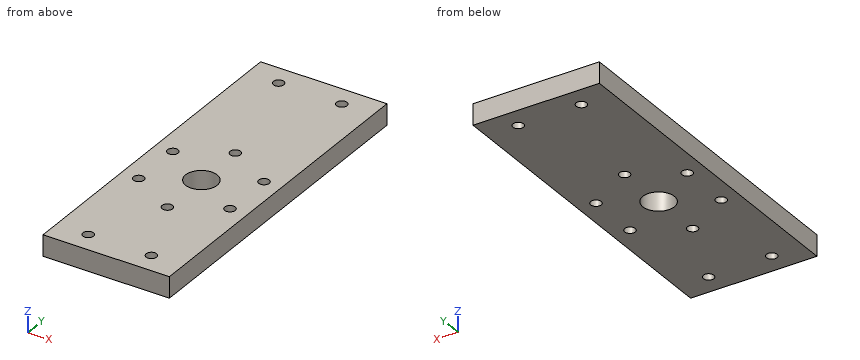
```python
from build123d import *

# Parameters (mm, degrees)
SKETCH1_W           = 76.2
SKETCH1_H           = 203.2
BOSS_EXTRUDE1_DEPTH = 12.7
SKETCH2_R           = 3.175
CUT_EXTRUDE1_DEPTH  = 12.7
SKETCH3_R           = 9.525
CUT_EXTRUDE2_DEPTH  = 12.7
SKETCH4_R           = 3.175
CUT_EXTRUDE3_DEPTH  = 12.7


with BuildPart() as part:
    # Sketch1 → Boss-Extrude1 (new body)
    with BuildSketch(Plane.XY):
        with Locations((38.1, 101.6)):
            Rectangle(SKETCH1_W, SKETCH1_H)
    extrude(amount=BOSS_EXTRUDE1_DEPTH)

    # Sketch2 → Cut-Extrude1 (cut)
    with BuildSketch(Plane(origin=(0, 0, 0), x_dir=(-1, 0, 0), z_dir=(0, 0, -1))):
        with Locations((-57.15, 190.5)):
            Circle(SKETCH2_R)
        with Locations((-19.05, 190.5)):
            Circle(SKETCH2_R)
        with Locations((-19.05, 12.7)):
            Circle(SKETCH2_R)
        with Locations((-57.15, 12.7)):
            Circle(SKETCH2_R)
    extrude(amount=-CUT_EXTRUDE1_DEPTH, mode=Mode.SUBTRACT)

    # Sketch3 → Cut-Extrude2 (cut)
    with BuildSketch(Plane.XY.offset(12.7)):
        with Locations((38.1, 88.9)):
            Circle(SKETCH3_R)
    extrude(amount=-CUT_EXTRUDE2_DEPTH, mode=Mode.SUBTRACT)

    # Sketch4 → Cut-Extrude3 (cut)
    with BuildSketch(Plane.XY.offset(12.7)):
        with Locations((38.1, 120.65)):
            Circle(SKETCH4_R)
        with Locations((65.59630657, 104.775)):
            Circle(SKETCH4_R)
        with Locations((65.59630657, 73.025)):
            Circle(SKETCH4_R)
        with Locations((38.1, 57.15)):
            Circle(SKETCH4_R)
        with Locations((10.60369343, 73.025)):
            Circle(SKETCH4_R)
        with Locations((10.60369343, 104.775)):
            Circle(SKETCH4_R)
    extrude(amount=-CUT_EXTRUDE3_DEPTH, mode=Mode.SUBTRACT)


solid = part.part
```
Geometry: final body of the model. Coordinates: model frame, mm. Round coordinates to 2 decimals unless told otherwise and drop trailing zeros. Loops run counter-clockwise (first coordinate to the right, second up) from the corner with the lowest first, then second, coordinate; pieces in that order, holes last.
Item 1: Section C-C, the plane x = 38.1. Output: boundary loops of the cut face in (y, z) (3 decimals), plus the area to 3 significant figures.
Checked values:
outline: (0, 0) - (53.975, 0) - (53.975, 12.7) - (0, 12.7) - close; (60.325, 0) - (79.375, 0) - (79.375, 12.7) - (60.325, 12.7) - close; (98.425, 0) - (117.475, 0) - (117.475, 12.7) - (98.425, 12.7) - close; (123.825, 0) - (203.2, 0) - (203.2, 12.7) - (123.825, 12.7) - close
area: 2,180 mm2
Item 2: Contact query for a flat-ended pin moving along its axis: P1, Ø4, axis at x = 65.6, y = 73.03, coming from the +Z side. Output: stop coordinate, or through.
Checked values:
P1: passes through
Item 3: Section D-D, the plane y = 120.65. Output: boundary loops of the cut face in (x, z) (3 decimals), plus the area to 3 significant figures.
Checked values:
outline: (0, 0) - (34.925, 0) - (34.925, 12.7) - (0, 12.7) - close; (41.275, 0) - (76.2, 0) - (76.2, 12.7) - (41.275, 12.7) - close
area: 887 mm2
Item 4: Section B-B, the plane y = 190.5. Output: boundary loops of the cut face in (x, z) (3 decimals).
Checked values:
outline: (0, 0) - (15.875, 0) - (15.875, 12.7) - (0, 12.7) - close; (22.225, 0) - (53.975, 0) - (53.975, 12.7) - (22.225, 12.7) - close; (60.325, 0) - (76.2, 0) - (76.2, 12.7) - (60.325, 12.7) - close
Item 5: Line query: L1, parallel to Y at x = 38.1, z = 7.5 (3 decimals); L2, parallel to Y at x = 19.05, z = 8.25 (3 decimals); L3, parallel to Y at x = 11.5, z = 4. Output: solid intervals per line, ascending.
Checked values:
L1: y = 0 to 53.975, 60.325 to 79.375, 98.425 to 117.475, 123.825 to 203.2
L2: y = 0 to 9.525, 15.875 to 187.325, 193.675 to 203.2
L3: y = 0 to 69.98, 76.07 to 101.73, 107.82 to 203.2
Item 6: Section A-A, the plane x = 57.15. Output: boundary loops of the cut face in (y, z) (3 decimals).
Checked values:
outline: (0, 0) - (9.525, 0) - (9.525, 12.7) - (0, 12.7) - close; (15.875, 0) - (187.325, 0) - (187.325, 12.7) - (15.875, 12.7) - close; (193.675, 0) - (203.2, 0) - (203.2, 12.7) - (193.675, 12.7) - close
